Geometry check sheet. Reference: the model listing, model coordinates, mm. A direction names the side the tool comes from. Coordinates: 2 decimals unless noted, no trailing zeros. Write each loop counter-clockwise with the first axis right and the second up, starting at its lowest first coordinate (ties: lowest second). Pieces come first, ordered by that corner, then holes. Notation, with made-up numbers: (65.25, 28.25) -> (79.25, 28.25) arc R23 ccw to (79.25, 44.25) -> close; hole circle Ø8 at (19, -39.5). An arc over 180 degrees is marked (long way). Answer in a Markdown table with one row per item. Add a question column.
Q1. Release check for a two-part mould opening along X. For faces 1 (the face through (0, 3, -2.094)), 2 (the face through (-1, 3, 12.116)), 3 (the face through (-14, -4, -18)), 4 (the face through (13, 2, 19)) record: pulls with the +X half, pulls with the -X half, needs draft (parallel to the pull), parting line crosses it, or undercut.
Q2. Section check A-A, the plane x = 7.5. Record the boundary of the cut face in (y, z).
Q3. Section check B-B, the plane z = 14. Record the boundary of the cut face in (x, y).
Q4. Tool access check on faces 5 (the face through (14, -5, 18)), 6 (the face through (-3, 3, -0.31)), 7 (the face through (0, 0, 7)). Record the directions out of +Z, -Z, +X, -X, +Y, -Y that give a thin tool (end or side, any length) a straight path to the whole face; none if there is none.
Q5. Thickness scan on line 1 (X direction, y = 0.7, z = 14); line 2 (Z direction, x = -7.5, y = 1.4); line 3 (Y direction, x = -4.5, z = 3). Record the ranges inside material, lowest first.
Q6. Gauge pin test, flat ends, axial feed: P1, Ø1.7, axis at x = 3.5, y = -1, coming from the +Z side; P2, Ø3, axis at x = -7.5, z = 14, coming from the +Y side; P3, Ø5.5, axis at x = -7.5, z = 14, coming from the +Y side. Record the tip position at first contact, or that the pin passes through.
Q7. Section check C-C, the plane y = -4.5. Record the boundary of the cut face in (x, z), and give its area (3 significant figures).
```python
from build123d import *

# Parameters (mm, degrees)
BOSS_EXTRUDE1_DEPTH                                 = 4.25
BOSS_EXTRUDE2_DEPTH                                 = 30
FILLET1_R                                           = 5
CSK_FOR_M3_COUNTERSUNK_FLAT_HEAD_SCREW1_D           = 3.4
CSK_FOR_M3_COUNTERSUNK_FLAT_HEAD_SCREW1_CSINK_D     = 6.3
CSK_FOR_M3_COUNTERSUNK_FLAT_HEAD_SCREW1_CSINK_ANGLE = 90
CUT_EXTRUDE3_DEPTH                                  = 2


with BuildPart() as part:
    # Sketch1 → Boss-Extrude1 (new body)
    with BuildSketch(Plane(origin=(0, 0, 0), x_dir=(1, 0, 0), z_dir=(0, 1, 0))):
        with BuildLine():
            Line((15, 15), (15, 20))
            Line((15, 20), (10, 20))
            Line((10, 20), (-10, 20))
            ThreePointArc((-10, 20), (-13.535533906, 18.535533906), (-15, 15))
            Line((-15, 15), (-15, -15))
            ThreePointArc((-15, -15), (-13.535533906, -18.535533906), (-10, -20))
            Line((-10, -20), (10, -20))
            ThreePointArc((10, -20), (13.535533906, -18.535533906), (15, -15))
            Line((15, -15), (15, 15))
        make_face()
    extrude(amount=BOSS_EXTRUDE1_DEPTH)

    # Sketch8 → Boss-Extrude2 (add)
    with BuildSketch(Plane(origin=(15, 0, 0), x_dir=(0, 0, -1), z_dir=(1, 0, 0))):
        Polygon((4.788040489, 0), (20, 0), (20, -7.65), (5.253900522, -7.65), (-20, -7.65), (-20, -3.4), (4.788040489, -3.4), align=None)
    extrude(amount=-BOSS_EXTRUDE2_DEPTH)

    # Fillet1
    fillet1_edges = [part.edges().sort_by_distance(p)[0] for p in [
        (-15, -5.525, 20),
        (15, -5.525, 20),
        (-15, -3.825, -20),
        (15, -1.7, -20),
    ]]
    fillet(fillet1_edges, radius=FILLET1_R)

    # CSK for M3 Countersunk Flat Head Screw1 (through all)
    with Locations(Plane(origin=(7.5, 4.25, 14), x_dir=(0, 0, 1), z_dir=(0, 1, 0))):
        with Locations((0, 0), (0, -15)):
            CounterSinkHole(CSK_FOR_M3_COUNTERSUNK_FLAT_HEAD_SCREW1_D / 2, CSK_FOR_M3_COUNTERSUNK_FLAT_HEAD_SCREW1_CSINK_D / 2, counter_sink_angle=CSK_FOR_M3_COUNTERSUNK_FLAT_HEAD_SCREW1_CSINK_ANGLE)

    # Sketch16 → Cut-Extrude3 (cut)
    with BuildSketch(Plane(origin=(0, 4.25, 0), x_dir=(1, 0, 0), z_dir=(0, 1, 0))):
        with BuildLine():
            Line((-4.458875061, 2.093953282), (-4.458875061, 0.309949228))
            Line((-4.458875061, 0.309949228), (-0.672122679, 0.309949228))
            Line((-0.672122679, 0.309949228), (-0.672122679, -0.295533742))
            add(Edge.make_bspline(
                [(-0.672122679, -0.295533742), (-0.672504144, -0.346007588), (-0.673250223, -0.444725636), (-0.687535915, -0.588091446), (-0.711269814, -0.723049373), (-0.748906576, -0.848005309), (-0.795186736, -0.964950699), (-0.856795731, -1.071025204), (-0.926036377, -1.170327836), (-1.010647749, -1.259432456), (-1.109289731, -1.34061223), (-1.221698501, -1.418754612), (-1.353111911, -1.488366917), (-1.500999377, -1.552487837), (-1.66430924, -1.614037158), (-1.844048215, -1.67060951), (-2.041510814, -1.718785961), (-2.179182831, -1.747242983), (-2.25068209, -1.762021993)],
                knots=[0, 0, 0, 0, 0.000151354, 0.000296022, 0.000431716, 0.000561725, 0.000686937, 0.000808031, 0.00092887, 0.001049364, 0.001175264, 0.001311639, 0.001459344, 0.001620515, 0.001794996, 0.001982705, 0.00218542, 0.002404451, 0.002404451, 0.002404451, 0.002404451], degree=3))
            add(Edge.make_bspline(
                [(-2.25068209, -1.762021993), (-2.387123246, -1.789200508), (-2.648649934, -1.841295546), (-3.023584407, -1.921428366), (-3.362673147, -2.002832785), (-3.666100231, -2.077858492), (-3.927379781, -2.154644362), (-4.146751884, -2.219240543), (-4.32008565, -2.279378782), (-4.417682148, -2.322811057), (-4.45961412, -2.341471572)],
                knots=[0, 0, 0, 0, 0.000417367, 0.000799998, 0.001150089, 0.001463532, 0.001737527, 0.001966934, 0.002149658, 0.002287303, 0.002287303, 0.002287303, 0.002287303], degree=3))
            Line((-4.45961412, -2.341471572), (-4.458875061, -4.175738487))
            add(Edge.make_bspline(
                [(-4.458875061, -4.175738487), (-4.402589194, -4.151927467), (-4.273325007, -4.097243897), (-4.049026625, -4.021563183), (-3.76980856, -3.944375115), (-3.44421419, -3.85993596), (-3.082911414, -3.77340803), (-2.69996289, -3.679173777), (-2.299298994, -3.5850796), (-2.02650801, -3.520868388), (-1.887209172, -3.488079375)],
                knots=[0, 0, 0, 0, 0.000183303, 0.000420968, 0.000709434, 0.001052273, 0.001430025, 0.001823964, 0.002235386, 0.002664705, 0.002664705, 0.002664705, 0.002664705], degree=3))
            add(Edge.make_bspline(
                [(-1.887209172, -3.488079375), (-1.773168942, -3.460587046), (-1.5527428, -3.40744766), (-1.242137194, -3.301932392), (-0.961961493, -3.180824272), (-0.712628496, -3.043118308), (-0.494327391, -2.883770123), (-0.309294243, -2.700614679), (-0.160659908, -2.489955128), (-0.089741414, -2.335127445), (-0.054041414, -2.257187997)],
                knots=[0, 0, 0, 0, 0.000351778, 0.000679945, 0.00098268, 0.001266475, 0.001532679, 0.001790935, 0.002044255, 0.002301038, 0.002301038, 0.002301038, 0.002301038], degree=3))
            Line((-0.054041414, -2.257187997), (-0.017001018, -2.256815895))
            add(Edge.make_bspline(
                [(-0.017001018, -2.256815895), (0.029911866, -2.365823451), (0.123313913, -2.582853997), (0.323884915, -2.877351795), (0.561124066, -3.147418036), (0.791801521, -3.347016191), (0.996667391, -3.486871195), (1.159796885, -3.579888369), (1.331125187, -3.659692635), (1.511272618, -3.724161338), (1.699423762, -3.777423006), (1.896777905, -3.815590183), (2.10218195, -3.840681678), (2.242029099, -3.845564971), (2.31292232, -3.848040477)],
                knots=[0, 0, 0, 0, 0.000355311, 0.000707414, 0.001063218, 0.001431749, 0.001618768, 0.001806724, 0.001994483, 0.002185005, 0.002380132, 0.002580552, 0.002787459, 0.003000185, 0.003000185, 0.003000185, 0.003000185], degree=3))
            add(Edge.make_bspline(
                [(2.31292232, -3.848040477), (2.385587327, -3.843063086), (2.528387107, -3.833281621), (2.736157027, -3.804081983), (2.934377079, -3.769477794), (3.12157362, -3.72614897), (3.298551, -3.672971002), (3.465300172, -3.611887222), (3.621747563, -3.542152622), (3.767015737, -3.462240208), (3.901655002, -3.374411599), (4.028165561, -3.280431232), (4.139686737, -3.173179002), (4.245201989, -3.061210534), (4.337161514, -2.937791912), (4.421171972, -2.806974416), (4.492481699, -2.666595654), (4.572833747, -2.470528249), (4.655111908, -2.221765184), (4.747022893, -1.928865862), (4.815938639, -1.640339407), (4.873772811, -1.360763019), (4.911134187, -1.087285562), (4.938041391, -0.821456672), (4.942448373, -0.562034079), (4.934759857, -0.391801423), (4.930980872, -0.308130323)],
                knots=[0, 0, 0, 0, 0.000218439, 0.000429273, 0.000629045, 0.000821988, 0.00100531, 0.001183082, 0.001354416, 0.001518656, 0.001679866, 0.001836496, 0.001990536, 0.002143381, 0.002297551, 0.002451481, 0.002609328, 0.002769115, 0.003086745, 0.003395031, 0.003689736, 0.003976245, 0.004251139, 0.004517418, 0.004777346, 0.005028594, 0.005028594, 0.005028594, 0.005028594], degree=3))
            add(Edge.make_bspline(
                [(4.930980872, -0.308130323), (4.928380241, -0.083891229), (4.92331038, 0.353257086), (4.887880892, 0.889981636), (4.849888886, 1.296449232), (4.81849973, 1.578640143), (4.783827219, 1.842751715), (4.756374827, 2.012069012), (4.743098736, 2.093951568)],
                knots=[0, 0, 0, 0, 0.000672659, 0.001311332, 0.001612904, 0.001897366, 0.002163083, 0.002411927, 0.002411927, 0.002411927, 0.002411927], degree=3))
            Line((4.743098736, 2.093951568), (-4.458875061, 2.093953282))
        make_face()
        with BuildLine():
            add(Edge.make_bspline(
                [(3.524901679, 0.309949228), (3.5362357, 0.265056815), (3.562459702, 0.161187345), (3.581770379, -0.022092437), (3.596059535, -0.251690395), (3.596338527, -0.421053384), (3.596490933, -0.513571537)],
                knots=[0, 0, 0, 0, 0.000138759, 0.000321052, 0.000551505, 0.00082896, 0.00082896, 0.00082896, 0.00082896], degree=3))
            add(Edge.make_bspline(
                [(3.596490933, -0.513571537), (3.597082169, -0.601000244), (3.598262348, -0.775518572), (3.546964591, -1.035855351), (3.4603018, -1.291694822), (3.357800432, -1.499038994), (3.250131892, -1.654091538), (3.148195375, -1.757518057), (3.02726046, -1.845102985), (2.888483977, -1.920565561), (2.729515001, -1.975864581), (2.554400178, -2.022986207), (2.359997891, -2.051855745), (2.224042634, -2.059862294), (2.153134709, -2.064038137)],
                knots=[0, 0, 0, 0, 0.000261725, 0.000522434, 0.000791185, 0.001070744, 0.001213016, 0.001355807, 0.001504013, 0.001659567, 0.001827887, 0.002007617, 0.002203059, 0.002416111, 0.002416111, 0.002416111, 0.002416111], degree=3))
            add(Edge.make_bspline(
                [(2.153134709, -2.064038137), (2.098038917, -2.062071411), (1.990380235, -2.058228374), (1.833615321, -2.036444408), (1.684147968, -2.004273349), (1.544949695, -1.954070069), (1.412062778, -1.894607052), (1.289839735, -1.818968912), (1.176559769, -1.72966981), (1.070777099, -1.630128202), (0.976208078, -1.517460335), (0.892824958, -1.394333332), (0.82440131, -1.258660147), (0.766734521, -1.113542778), (0.720573152, -0.95726533), (0.688091814, -0.790869848), (0.666338768, -0.613623823), (0.662560413, -0.491981725), (0.660613067, -0.429287962)],
                knots=[0, 0, 0, 0, 0.000165289, 0.000322979, 0.000474201, 0.000623029, 0.000766025, 0.000910277, 0.001052884, 0.001198201, 0.001345237, 0.001493286, 0.00164328, 0.001800117, 0.00196124, 0.002131355, 0.002308205, 0.002496292, 0.002496292, 0.002496292, 0.002496292], degree=3))
            Line((0.660613067, -0.429287962), (0.66236726, 0.309949228))
            Line((0.66236726, 0.309949228), (3.524901679, 0.309949228))
        make_face(mode=Mode.SUBTRACT)
        Polygon((-0.236655826, -5.03436712), (-1.34639128, -5.03436712), (-1.34639128, -8.020075729), (-4.477744211, -8.020075729), (-4.477744211, -9.129811183), (-1.34639128, -9.129811183), (-1.34639128, -12.115519792), (-0.236655826, -12.115519792), (-0.236655826, -9.129811183), (2.870423051, -9.129811183), (2.870423051, -8.020075729), (-0.236655826, -8.020075729), align=None)
    extrude(amount=-CUT_EXTRUDE3_DEPTH, mode=Mode.SUBTRACT)


solid = part.part
```
Calculated:
| question | item | result |
|---|---|---|
| 1 | face 1 | undercut |
| 1 | face 2 | undercut |
| 1 | face 3 | pulls with the -X half |
| 1 | face 4 | pulls with the +X half |
| 2 | outline | (-7.65, -20) -> (4.25, -20) -> (4.25, 10.85) -> (2.8, 12.3) -> (0, 12.3) -> (0, -4.79) -> (-3.4, -4.79) -> (-3.4, 12.3) -> (-7.65, 12.3) -> close; (-7.65, 15.7) -> (-3.4, 15.7) -> (-3.4, 20) -> (-7.65, 20) -> close; (0, 15.7) -> (2.8, 15.7) -> (4.25, 17.15) -> (4.25, 20) -> (0, 20) -> close |
| 3 | outline | (-15, -7.65) -> (-9.2, -7.65) -> (-9.2, -3.4) -> (-15, -3.4) -> close; (-15, 0) -> (-9.2, 0) -> (-9.2, 2.8) -> (-10.65, 4.25) -> (-15, 4.25) -> close; (-5.8, -7.65) -> (5.8, -7.65) -> (5.8, -3.4) -> (-5.8, -3.4) -> close; (-5.8, 0) -> (5.8, 0) -> (5.8, 2.8) -> (4.35, 4.25) -> (-4.35, 4.25) -> (-5.8, 2.8) -> close; (9.2, -7.65) -> (15, -7.65) -> (15, -3.4) -> (9.2, -3.4) -> close; (9.2, 0) -> (15, 0) -> (15, 4.25) -> (10.65, 4.25) -> (9.2, 2.8) -> close |
| 4 | face 5 | +Z, +X, +Y, -Y |
| 4 | face 6 | +Y |
| 4 | face 7 | +Z, +X, -X |
| 5 | line 1 | x = -15 to -9.2, -5.8 to 5.8, 9.2 to 15 |
| 5 | line 2 | z = -20 to 12.3, 15.7 to 20 |
| 5 | line 3 | y = -7.65 to -3.4, 0 to 4.25 |
| 6 | P1 | stops at z = -4.79 |
| 6 | P2 | passes through |
| 6 | P3 | stops at y = 3.85 |
| 7 | outline | (-15, -15) arc R5 ccw to (-10, -20) -> (10, -20) arc R5 ccw to (15, -15) -> (15, 15) arc R5 ccw to (10, 20) -> (-10, 20) arc R5 ccw to (-15, 15) -> close; hole circle Ø3.4 at (-7.5, 14); hole circle Ø3.4 at (7.5, 14) |
| 7 | area | 1,160 mm² |
